Verification items for this drawing (mm, ordinates from the low corner). Coordinates: 2 decimals unless noted, no trailing zeros. Write each loop counter-clockwise with the first axis right and the second up, starting at its lowest first coordinate (ties: lowest second). Pieces come first, ordered by that corner, then holes.
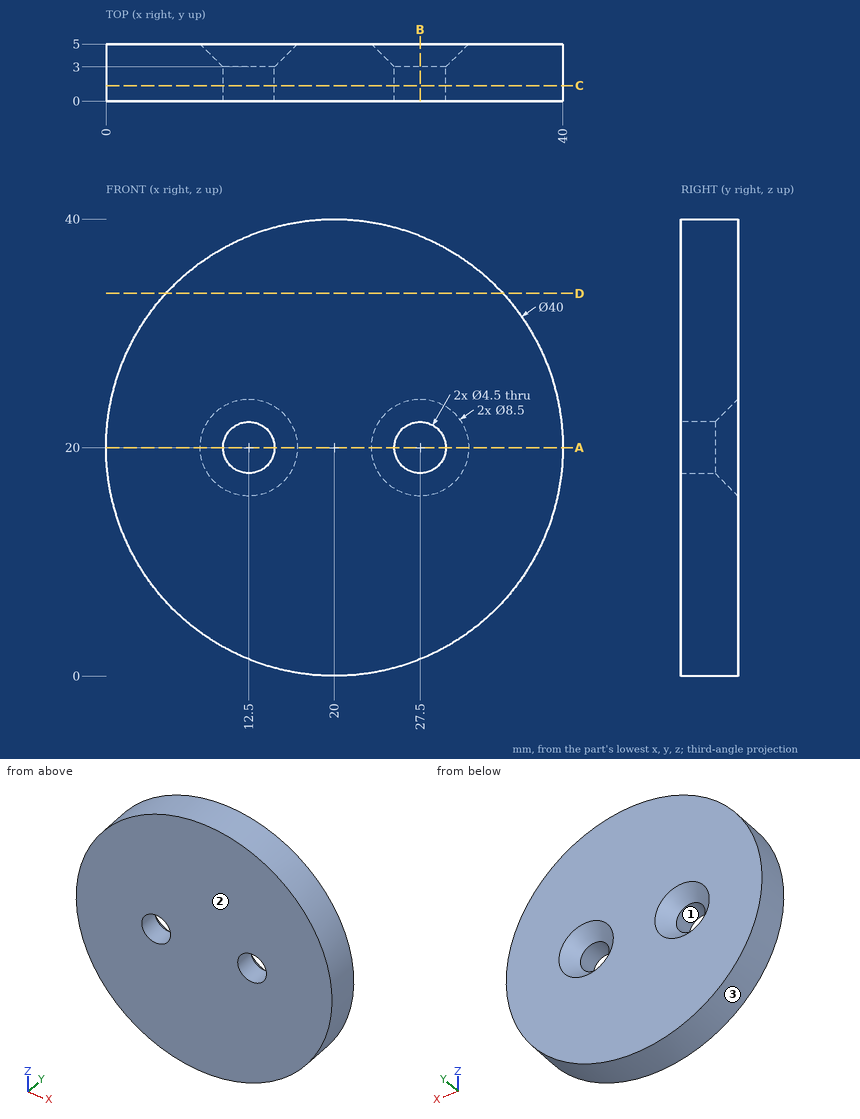
1. Gauge pin test, flat ends, axial feed: pin 1 Ø1 at (x, y) = (21.5, 3.5) entering from +Z (3 decimals); pin 2 Ø5 at (x, z) = (12.5, 20) entering from +Y. Record the tip position at first contact, or that the pin passes through.
Computed values:
pin 1: stops at z = 39.975
pin 2: stops at y = 3.25
2. Sectioned sample at D-D, the plane z = 33.5. Record the boundary of the cut face in (x, y).
Computed values:
outline: (5.24, 0) - (34.76, 0) - (34.76, 5) - (5.24, 5) - close
3. Thickness scan on line 1 along X through (y, z) = (1.45, 20); line 2 along X through (y, z) = (2.25, 18); line 3 along X through (y, z) = (2.8, 7.5). Record the ranges inside material, lowest first.
Computed values:
line 1: x = 0 to 10.25, 14.75 to 25.25, 29.75 to 40
line 2: x = 0.1 to 11.47, 13.53 to 26.47, 28.53 to 39.9
line 3: x = 4.39 to 35.61
4. Sectioned sample at A-A, the plane z = 20. Record the boundary of the cut face in (x, y).
Computed values:
outline: (0, 0) - (10.25, 0) - (10.25, 3) - (8.25, 5) - (0, 5) - close; (14.75, 0) - (25.25, 0) - (25.25, 3) - (23.25, 5) - (16.75, 5) - (14.75, 3) - close; (29.75, 0) - (40, 0) - (40, 5) - (31.75, 5) - (29.75, 3) - close
5. Sectioned sample at B-B, the plane x = 27.5. Record the boundary of the cut face in (y, z).
Computed values:
outline: (0, 1.46) - (5, 1.46) - (5, 15.75) - (3, 17.75) - (0, 17.75) - close; (0, 22.25) - (3, 22.25) - (5, 24.25) - (5, 38.54) - (0, 38.54) - close
6. Sectioned sample at C-C, the plane y = 1.35. Record the boundary of the cut face in (x, z).
Computed values:
outline: circle Ø40 at (20, 20); hole circle Ø4.5 at (12.5, 20); hole circle Ø4.5 at (27.5, 20)
7. Draft check along X on the marked faces 1, 2 and 3. Enter one of: released by +X, released by -X, zero draft, split by the parting line, or undercut.
Computed values:
face 1: undercut
face 2: zero draft
face 3: split by the parting line
